```python
from build123d import *

# Parameters (mm, degrees)
F0_W           = 101.6
F0_H           = 19.05
F1_DEPTH       = 6.35
F3_D           = 6.7564
F3_CSINK_D     = 13.4874
F3_CSINK_ANGLE = 82
F4_R           = 6.35


with BuildPart() as f1:
    # F0 (on Front) → F1 (new body)
    with BuildSketch(Plane.XZ):
        Rectangle(F0_W, F0_H)
    extrude(amount=F1_DEPTH)

    # F3 (through all)
    with Locations(Plane.XZ.offset(6.35)):
        with Locations((-41.275, 0), (41.275, 0)):
            CounterSinkHole(F3_D / 2, F3_CSINK_D / 2, counter_sink_angle=F3_CSINK_ANGLE)

    # F4
    f4_edges = [f1.edges().sort_by_distance(p)[0] for p in [
        (-50.8, -3.175, 9.525),
        (-50.8, -3.175, -9.525),
        (50.8, -3.175, -9.525),
        (50.8, -3.175, 9.525),
    ]]
    fillet(f4_edges, radius=F4_R)


solid = f1.part
```
Work out the finished part from the listing and answer in its coordinate system (mm). Give positions to 0.01 mm unless a question says otherwise; leave off trailing zeros. Write each loop counter-clockwise with the first axis right and the second up, starting at its lowest first coordinate (ties: lowest second). Pieces come first, ordered by that corner, then holes.
(1) The part is cut by section A-A on z = 0. Write down the section's boundary in (x, y).
Final values:
outline: (-50.8, -6.35) - (-48.02, -6.35) - (-44.65, -2.48) - (-44.65, 0) - (-50.8, 0) - close; (-37.9, -2.48) - (-34.53, -6.35) - (34.53, -6.35) - (37.9, -2.48) - (37.9, 0) - (-37.9, 0) - close; (44.65, -2.48) - (48.02, -6.35) - (50.8, -6.35) - (50.8, 0) - (44.65, 0) - close
(2) Straight lines are drawn through the part: line 1 (X direction, y = -0.7, z = 0); line 2 (X direction, y = -1.25, z = 1); line 3 (Z direction, x = 44, y = -1) (3 decimals). For each, find the intervals that lie inside material, in ascending order.
Final values:
line 1: x = -50.8 to -44.65, -37.9 to 37.9, 44.65 to 50.8
line 2: x = -50.8 to -44.5, -38.05 to 38.05, 44.5 to 50.8
line 3: z = -9.525 to -1.997, 1.997 to 9.525
(3) The part is cut by section B-B on y = -1.5. Write down the section's boundary in (x, z) (3 decimals), plus the area to 3 significant figures.
Final values:
outline: (-50.8, -3.175) arc R6.35 ccw to (-44.45, -9.525) - (44.45, -9.525) arc R6.35 ccw to (50.8, -3.175) - (50.8, 3.175) arc R6.35 ccw to (44.45, 9.525) - (-44.45, 9.525) arc R6.35 ccw to (-50.8, 3.175) - close; hole circle Ø6.756 at (-41.275, 0); hole circle Ø6.756 at (41.275, 0)
area: 1,830 mm2
(4) Flat-ended cylindrical pins translate along their axes: pin 1 Ø5.5 at (x, z) = (41.275, 0) entering from +Y; pin 2 Ø3 at (y, z) = (-4, -7.5) entering from +X. Find the tip coordinate at first contact, or state that the pin passes through.
Final values:
pin 1: passes through
pin 2: stops at x = 50.14
